Design review of the part built by this model. Coordinates are the model's own, in mm. A direction names the side the tool comes from. Give positions to 0.01 mm unless a question says otherwise; leave off trailing zeros. Order: outer loops, then holes, each group sorted by start corner. A loop starts at its lowest first (then second) coordinate and runs counter-clockwise, first axis right, second up. Notation, with made-up numbers: (-18.5, 46.25) -> (27.5, 46.25) arc R18 cw to (27.5, 69.25) -> close; hole circle Ø2 at (87, 8.5). An arc over 180 degrees is marked (long way). Return JSON: item names as keys, results as strings.
```python
from build123d import *

# Parameters (mm, degrees)
SKETCH2_W                       = 120
SKETCH2_H                       = 50
BOSS_EXTRUDE1_DEPTH             = 15
SKIZZE7_R                       = 1.5
SCHNITT_LINEAR_AUSTRAGEN6_DEPTH = 10
SKIZZE10_W                      = 12.5
SKIZZE10_H                      = 1.5
ROTATION3_ANGLE                 = 180
SKIZZE11_W                      = 12.5
SKIZZE11_H                      = 1.5
ROTATION4_ANGLE                 = 180
SKIZZE12_R                      = 2
SCHNITT_LINEAR_AUSTRAGEN7_DEPTH = 83.233536557
SKIZZE13_W                      = 15
SKIZZE13_H                      = 10
SCHNITT_LINEAR_AUSTRAGEN8_DEPTH = 126.771499808


with BuildPart() as part:
    # Sketch2 → Boss-Extrude1 (new body)
    with BuildSketch(Plane(origin=(0, 0, 0), x_dir=(1, 0, 0), z_dir=(0, 1, 0))):
        with Locations((13.101876656, 9.54663752)):
            Rectangle(SKETCH2_W, SKETCH2_H)
    extrude(amount=BOSS_EXTRUDE1_DEPTH)

    # Skizze7 → Schnitt-Linear austragen6 (cut)
    with BuildSketch(Plane.ZY.offset(46.898123344)):
        with Locations((-9.54663752, 2.5)):
            Circle(SKIZZE7_R)
    extrude(amount=-SCHNITT_LINEAR_AUSTRAGEN6_DEPTH, mode=Mode.SUBTRACT)

    # Sketch3 → Schnitt-Rotation1 (revolve, cut)
    with BuildSketch(Plane(origin=(0, 0, 0), x_dir=(1, 0, 0), z_dir=(0, 1, 0))):
        Polygon((63.101876656, 9.54663752), (63.101876656, 17.04663752), (3.101876656, 17.04663752), (3.101876656, 19.54663752), (-36.898123344, 19.54663752), (-36.898123344, 9.54663752), align=None)
    revolve(axis=Axis((74.354835368, 0, -9.54663752), (-1, 0, 0)), mode=Mode.SUBTRACT)

    # Skizze10 → Rotation3 (revolve)
    with BuildSketch(Plane.XZ):
        with Locations((46.851876656, -16.29663752)):
            Rectangle(SKIZZE10_W, SKIZZE10_H)
    revolve(axis=Axis((85.744816074, 0, -9.54663752), (1, 0, 0)), revolution_arc=ROTATION3_ANGLE)

    # Skizze11 → Rotation4 (revolve)
    with BuildSketch(Plane.XZ):
        with Locations((21.851876656, -16.29663752)):
            Rectangle(SKIZZE11_W, SKIZZE11_H)
    revolve(axis=Axis((95.037830494, 0, -9.54663752), (1, 0, 0)), revolution_arc=ROTATION4_ANGLE)

    # Skizze12 → Schnitt-Linear austragen7 (cut, through all)
    with BuildSketch(Plane.XZ):
        with Locations(Location((-39.398123344, 7.95336248, 0), (0, 0, 270))):
            Circle(SKIZZE12_R)
        with Locations(Location((13.101876656, 7.95336248, 0), (0, 0, 270))):
            Circle(SKIZZE12_R)
        with Locations(Location((65.601876656, 7.95336248, 0), (0, 0, 270))):
            Circle(SKIZZE12_R)
    schnitt_linear_austragen7 = extrude(amount=-SCHNITT_LINEAR_AUSTRAGEN7_DEPTH, mode=Mode.SUBTRACT)

    # Spiegeln1: Schnitt-Linear austragen7 across plane
    add(schnitt_linear_austragen7.mirror(Plane.XY.offset(-9.54663752)), mode=Mode.SUBTRACT)

    # Skizze13 → Schnitt-Linear austragen8 (cut, through all)
    with BuildSketch(Plane.ZY.offset(46.898123344)):
        with Locations((7.95336248, 10)):
            Rectangle(SKIZZE13_W, SKIZZE13_H)
        with Locations((-27.04663752, 10)):
            Rectangle(SKIZZE13_W, SKIZZE13_H)
    extrude(amount=-SCHNITT_LINEAR_AUSTRAGEN8_DEPTH, mode=Mode.SUBTRACT)


solid = part.part
```
Item 1: For pin 1 (5 mm diameter, centred on x = 36.5, z = 9, fed in from +Y); pin 2 (1 mm diameter, centred on x = 21.5, y = 9.5, fed in from +Z); pin 3 (8 mm diameter, centred on x = 35, y = 13, fed in from -Z), all flat-tipped, find the tip position at first contact; note any pin that passes through.
Result set:
{"pin 1": "stops at y = 5", "pin 2": "stops at z = 0.45", "pin 3": "stops at z = -19.55"}
Item 2: Wall thickness on L1, parallel to X at y = 4, z = -27; L2, parallel to X at y = 0.5, z = -5.5; L3, parallel to X at y = 3, z = -27.5: over which ranges is each line inside the solid? List them lowest first. Write a range as [from, to].
Result set:
{"L1": "x = [-46.9, -41.4], [-37.4, 11.1], [15.1, 63.6], [67.6, 73.1]", "L2": "x = [-46.9, -36.9], [63.1, 73.1]", "L3": "x = [-46.9, -41.35], [-37.45, 11.15], [15.05, 63.65], [67.55, 73.1]"}
Item 3: Machinability: for faces 1 (the face through (9.3, 7.5, -9.4)), 2 (the face through (-41.968, 1.036, -9.872)), 3 (the face through (12, 5, 5)), which of the approach directions +Z, -Z, +X, -X, +Y, -Y give a long, thin tool a straight path to every point of the face, cutting with its end or side? Answer none if there is none.
Result set:
{"face 1": "-Y", "face 2": "-X", "face 3": "+Z, +X, -X, +Y"}
Item 4: Add section B-B (x = 47.5). Give the boundary of the cut face in (y, z), plus the area to 3 significant figures.
Result set:
{"outline": "(0, -34.55) -> (5, -34.55) -> (5, -19.55) -> (15, -19.55) -> (15, 0.45) -> (5, 0.45) -> (5, 15.45) -> (0, 15.45) -> (0, -3.55) arc R6 cw to (0, -15.55) -> close", "area": "393 mm^2"}
Item 5: Add section C-C (z = -21). Give the boundary of the cut face in (x, y).
Result set:
{"outline": "(-46.9, 0) -> (73.1, 0) -> (73.1, 5) -> (-46.9, 5) -> close"}
Item 6: Mouldability with a two-part tool opening along Z and no side actions: class faces 4 (the face through (58, 7.5, -9.4)), 5 (the face through (12, 10, -19.547)), 6 (the face through (-46.898, 6, -9)) as released by +Z, released by -Z, zero draft, split by the parting line, or undercut.
Result set:
{"face 4": "undercut", "face 5": "released by -Z", "face 6": "zero draft"}
Item 7: Add section A-A (x = 32). Give the boundary of the cut face in (y, z).
Result set:
{"outline": "(0, -34.55) -> (5, -34.55) -> (5, -19.55) -> (15, -19.55) -> (15, 0.45) -> (5, 0.45) -> (5, 15.45) -> (0, 15.45) -> (0, -2.05) arc R7.5 cw to (0, -17.05) -> close"}
Item 8: Add section D-D (y = 2.5). Give the number of separate pieces and of enclosed holes in the cut face, plus the area to 3 significant figures.
Result set:
{"separate pieces": "1", "enclosed holes": "6", "area": "4,350 mm^2"}
